The listing builds one solid part. Answer for the finished solid, in the listing's coordinates (mm). A direction names the side the tool comes from. Round coordinates to 2 decimals unless told otherwise and drop trailing zeros. Write each loop counter-clockwise with the first axis right and the second up, starting at its lowest first coordinate (ties: lowest second). Pieces come first, ordered by that corner, then holes.
Item 1: Find section B-B on y = 15. Give the vertices of the cut face in (x, z), then the cut area to 3 significant figures.
Item 2: A tool of negligible diameter and unlimited length cuts with its end or side. For faces 5 (the face through (-14.413, 43.383, 2.465)), 6 (the face through (28, 78.785, 2)), 7 (the face through (0, 5, 2)), 8 (the face through (-28, 78.785, 2)), from which of +Z, -Z, +X, -X, +Y, -Y can it reach the whole face along a straight path? Write none if from no direction.
Item 3: Find section A-A on z = 4.05. Give the vertices of the cut face in (x, y), then the cut area to 3 significant figures.
Item 4: Each of these flat-tipped pins is pushed along its axis until it touches: pin 1 (1.5 mm diameter, centred on x = -3.5, z = 2.5, fed in from +Y); pin 2 (1.5 mm diameter, centred on y = 61, z = 3, fed in from -X); pin 3 (1.5 mm diameter, centred on y = 3.5, z = 2.5, fed in from +X). Where does it stop, or does it pass through?
Item 5: Find section D-D on x = 17.5. Give the vertices of the cut face in (y, z).
Item 6: Find the intervals of material crossed by probe 1 along X at (y, z) = (14, 4.5); probe 2 along Y at (x, z) = (-3.5, 0.75); probe 3 along X at (y, z) = (29, 0.9), in increasing order.
Item 7: Find section C-C on x = -0.5. Give the vertices of the cut face in (y, z), then the cut area to 3 significant figures.
Item 8: For a pull along X with two mould halves and no side action, classify faces 1 (the face through (-31.892, 80, 2)), 2 (the face through (2.6, 3, 2)), 3 (the face through (-2.6, 2, 2)), 4 (the face through (-14, 38, 0)) as +X half, -X half, draft (parallel to the pull), parting line (faces both ways), or undercut.
```python
from build123d import *

# Parameters (mm, degrees)
F1_DEPTH    = 5
F2_T1_DEPTH = 28.770290161


# Not quite as in the source:
# - a fillet or chamfer that OpenCascade refuses, or shapes differently, is made with other operations: its cross-section is extruded or revolved along the edge and cut away or added


with BuildPart() as f1:
    # F0 (on Top) → F1 (new body)
    with BuildSketch(Plane.XY):
        Polygon((-10, 0), (-2.6, 0), (-2.6, 5), (0, 5), (2.6, 5), (2.6, 0), (10, 0), (23.8918542134, 78.784620241), (31.8918542134, 78.784620241), (31.8918542134, 81.784620241), (20.5755738699, 81.784620241), (20.5755738699, 78.3334689187), (8.4202014333, 9.3969262079), (3.4202014333, 9.3969262079), (0, 9.3969262079), (-8.4202014333, 9.3969262079), (-20.5755738699, 78.3334689187), (-20.5755738699, 81.784620241), (-31.8918542134, 81.784620241), (-31.8918542134, 78.784620241), (-23.8918542134, 78.784620241), align=None)
    extrude(amount=F1_DEPTH)

    # F2: fillet of radius 5 on 2 edges, made by hand

    # F2_s2 → F2_t1 (cut)
    with BuildSketch(Plane.XY.offset(-11.8851450805)):
        with BuildLine():
            ThreePointArc((-25.3296319021, 81.784620241), (-22.3923068766, 80.8308680948), (-20.5755738699, 78.3334689187))
            Line((-20.5755738699, 78.3334689187), (-20.5755738699, 81.784620241))
            Line((-20.5755738699, 81.784620241), (-25.3296319021, 81.784620241))
        make_face()
        with BuildLine():
            ThreePointArc((20.5755738699, 78.3334689187), (22.3923068766, 80.8308680948), (25.3296319021, 81.784620241))
            Line((25.3296319021, 81.784620241), (20.5755738699, 81.784620241))
            Line((20.5755738699, 81.784620241), (20.5755738699, 78.3334689187))
        make_face()
    extrude(amount=F2_T1_DEPTH, mode=Mode.SUBTRACT)


solid = f1.part
```
Check values:
1. outline: (-12.64, 0) - (-9.41, 0) - (-9.41, 5) - (-12.64, 5) - close; (9.41, 0) - (12.64, 0) - (12.64, 5) - (9.41, 5) - close
1. area: 32.4 mm2
2. face 5: +Z, -Z, +Y
2. face 6: +Z, -Z, +X, -Y
2. face 7: +Z, -Z, -Y
2. face 8: +Z, -Z, -X, -Y
3. outline: (-31.89, 78.78) - (-23.89, 78.78) - (-10, 0) - (-2.6, 0) - (-2.6, 5) - (2.6, 5) - (2.6, 0) - (10, 0) - (23.89, 78.78) - (31.89, 78.78) - (31.89, 81.78) - (25.33, 81.78) arc R5 ccw to (20.58, 78.33) - (8.42, 9.4) - (-8.42, 9.4) - (-20.58, 78.33) arc R5 ccw to (-25.33, 81.78) - (-31.89, 81.78) - close
3. area: 686 mm2
4. pin 1: stops at y = 9.4
4. pin 2: stops at x = -20.89
4. pin 3: stops at x = 10.75
5. outline: (42.53, 0) - (60.89, 0) - (60.89, 5) - (42.53, 5) - close
6. probe 1: x = -12.47 to -9.23, 9.23 to 12.47
6. probe 2: y = 0 to 9.4
6. probe 3: x = -15.11 to -11.88, 11.88 to 15.11
7. outline: (5, 0) - (9.4, 0) - (9.4, 5) - (5, 5) - close
7. area: 22.0 mm2
8. face 1: -X half
8. face 2: undercut
8. face 3: undercut
8. face 4: draft
